The model under review builds one solid part; all positions refer to its coordinate system, in mm. A direction names the side the tool comes from. Round coordinates to 2 decimals unless told otherwise and drop trailing zeros. Write each loop counter-clockwise with the first axis right and the second up, starting at its lowest first coordinate (ties: lowest second). Pieces come first, ordered by that corner, then holes.
Item 1: Add section A-A (x = 0). Give the boundary of the cut face in (y, z), plus the area to 3 significant figures.
Item 2: To check wall thickness, follow L1, parallel to Z at x = 0, y = -22.5; L2, parallel to Z at x = 0, y = -17; L3, parallel to Y at x = 0, z = -12. State the ranges of each line that lie inside material, in increasing order.
Item 3: Machinability: for faces 4 (the face through (-4, -9, -15)), 5 (the face through (13, -18, -4)), which of the approach directions +Z, -Z, +X, -X, +Y, -Y give a long, thin tool a straight path to every point of the face, cutting with its end or side? Answer none if there is none.
Item 4: Add section B-B (z = 0). Give the boundary of the cut face in (x, y).
Item 5: Clearance check with flat-ended pins moving along their axes: pin 1 Ø2 at (y, z) = (-5, 8) entering from +X (3 decimals); pin 2 Ø6 at (x, y) = (-14.5, -6.5) entering from +Z; pin 3 Ø9 at (x, y) = (0, -9) entering from -Z; pin 4 Ø16 at (x, z) = (0, 0) entering from +Y. State where each tip first meets the part, or that it passes through.
Item 6: Add section D-D (y = -4). Give the boundary of the cut face in (x, z), plus the area to 3 significant figures.
Item 7: Draft analysis for pull direction Z (two halves, no side actions). For faces 1 (the face through (-9, 0, 5)), 2 (the face through (-1.302, -14.544, 9.915)), 3 (the face through (-4.336, -8.881, -19.524)), state which applies: +Z half, -Z half, draft (parallel to the pull), parting line (faces both ways), or undercut.
Item 8: Add section C-C (y = -23.5). Give the boundary of the cut face in (x, z).
```python
from build123d import *

# Parameters (mm, degrees)
F0_R     = 20
F0_R_2   = 10
F1_DEPTH = 18
F2_R     = 4
F3_DEPTH = 25
F4_R     = 13
F4_R_2   = 10
F5_DEPTH = 12
F6_SIZE  = 0.5


with BuildPart() as f1:
    # F0 (on Front) → F1 (new body)
    with BuildSketch(Plane.XZ):
        Circle(F0_R)
        Circle(F0_R_2, mode=Mode.SUBTRACT)
    extrude(amount=F1_DEPTH)

    # F2 (on Top) → F3 (cut)
    with BuildSketch(Plane.XY):
        with Locations((0, -9)):
            Circle(F2_R)
    extrude(amount=-F3_DEPTH, mode=Mode.SUBTRACT)

    # F4 (on face) → F5 (join)
    with BuildSketch(Plane.XZ.offset(18)):
        Circle(F4_R)
        Circle(F4_R_2, mode=Mode.SUBTRACT)
    extrude(amount=F5_DEPTH)

    # F6
    f6_edges = [f1.edges().sort_by_distance(p)[0] for p in [
        (-13, -30, 0),
        (-10, -30, 0),
        (-20, -18, 0),
        (-20, 0, 0),
    ]]
    chamfer(f6_edges, length=F6_SIZE)


solid = f1.part
```
Numbers:
1. outline: (-30, -12.5) - (-29.5, -13) - (-18, -13) - (-18, -19.5) - (-17.5, -20) - (-13, -20) - (-13, -10) - (-29.5, -10) - (-30, -10.5) - close; (-30, 10.5) - (-29.5, 10) - (0, 10) - (0, 19.5) - (-0.5, 20) - (-17.5, 20) - (-18, 19.5) - (-18, 13) - (-29.5, 13) - (-30, 12.5) - close; (-5, -20) - (-0.5, -20) - (0, -19.5) - (0, -10) - (-5, -10) - close
1. area: 351 mm2
2. L1: z = -13 to -10, 10 to 13
2. L2: z = -20 to -10, 10 to 20
2. L3: y = -30 to -13, -5 to 0
3. face 4: -Z
3. face 5: -Y
4. outline: (-20, -17.5) - (-19.5, -18) - (-13, -18) - (-13, -29.5) - (-12.5, -30) - (-10.5, -30) - (-10, -29.5) - (-10, 0) - (-19.5, 0) - (-20, -0.5) - close; (10, -29.5) - (10.5, -30) - (12.5, -30) - (13, -29.5) - (13, -18) - (19.5, -18) - (20, -17.5) - (20, -0.5) - (19.5, 0) - (10, 0) - close
5. pin 1: stops at x = 18.735
5. pin 2: stops at z = 16.36
5. pin 3: stops at z = -20
5. pin 4: passes through
6. outline: circle Ø40 at (0, 0); hole circle Ø20 at (0, 0)
6. area: 942 mm2
7. face 1: draft
7. face 2: undercut
7. face 3: parting line
8. outline: circle Ø26 at (0, 0); hole circle Ø20 at (0, 0)
